from build123d import *

# Parameters (mm, degrees)
F1_DEPTH = 25.4
F3_D     = 4.318
F3_DEPTH = 5.08
F3_TIP   = 1.2972580765
F5_D     = 2.9464
F5_DEPTH = 5.08
F5_TIP   = 0.885187864


with BuildPart() as f1:
    # F0 (on Front) → F1 (new body)
    with BuildSketch(Plane.XZ):
        with BuildLine():
            ThreePointArc((-3.175, 0), (-0.9299359697, 0.9299359697), (0, 3.175))
            Line((0, 3.175), (0, 31.75))
            Line((0, 31.75), (-3.175, 31.75))
            Line((-3.175, 31.75), (-3.175, 6.35))
            ThreePointArc((-3.175, 6.35), (-4.1049359697, 4.1049359697), (-6.35, 3.175))
            Line((-6.35, 3.175), (-22.225, 3.175))
            Line((-22.225, 3.175), (-22.225, 0))
            Line((-22.225, 0), (-3.175, 0))
        make_face()
    extrude(amount=F1_DEPTH)

    # F3
    with Locations(Plane(origin=(-3.175, 0, 0), x_dir=(0, -1, 0), z_dir=(-1, 0, 0))):
        with Locations((6.35, 12.7), (6.35, 25.4), (19.05, 25.4), (19.05, 12.7)):
            Hole(F3_D / 2, depth=F3_DEPTH)
            with Locations((0, 0, -(F3_DEPTH + F3_TIP / 2))):  # 118° drill point
                Cone(0, F3_D / 2, F3_TIP, mode=Mode.SUBTRACT)

    # F5
    with Locations(Plane(origin=(0, 0, 0), x_dir=(1, 0, 0), z_dir=(0, 0, -1))):
        with Locations((-6.35, 6.35), (-6.35, 19.05), (-15.875, 19.05), (-15.875, 6.35)):
            Hole(F5_D / 2, depth=F5_DEPTH)
            with Locations((0, 0, -(F5_DEPTH + F5_TIP / 2))):  # 118° drill point
                Cone(0, F5_D / 2, F5_TIP, mode=Mode.SUBTRACT)


solid = f1.part
Work out the finished part from the listing and answer in its coordinate system (mm). A direction names the side the tool comes from. Round coordinates to 2 decimals unless told otherwise and drop trailing zeros. Loops run counter-clockwise (first coordinate to the right, second up) from the corner with the lowest first, then second, coordinate; pieces in that order, holes last. Notation, with made-up numbers: (66, -10.5) - (71, -10.5) arc R20 cw to (71, 7.5) - close; hole circle Ø4 at (53.25, 75). An arc over 180 degrees is marked (long way). Use one line per item in the form item = value. Start each with the question number.
(1) Consider line 1 (Y direction, x = -6.35, z = 2); line 2 (Z direction, x = -0.9, y = -19.05); line 3 (Y direction, x = -1.75, z = 26.5). Determine where each line is inside the solid, lowest interval first.
(2) Find section C-C on y = -22.75. Determine the outline of the cut face in (x, z) (3 decimals).
(3) Which of the six approach directions +Z, -Z, +X, -X, +Y, -Y give full straight-line access (tool end or side, diameter ignored) to faces 1 (the face through (-17.28, -6.79, 1.61)), 2 (the face through (-14, -13, 3.175))?
(4) Find section D-D on x = -13.5. Determine the outline of the cut face in (y, z) (3 decimals).
(5) Flat-ended cylindrical pins translate along their axes: P1, Ø1.5, axis at x = -17.5, z = 4.5, coming from the +Y side; P2, Ø7, axis at y = -6.35, z = 12.7, coming from the -X side (3 decimals); P3, Ø3.5, axis at x = -15.875, y = -19.05, coming from the -Z side. Find the tip coordinate at first contact, or state that the pin passes through.
(6) Determine the mould class of faces 3 (the face through (-4.08, -12.52, 4.13)), 4 (the face through (-3.175, -13, 19)), 5 (the face through (-1.565, -19.518, 10.592)), 6 (the face through (-0.95, -12.52, 0.91)) for opening direction Z: +Z half, -Z half, draft (parallel to the pull), parting line (faces both ways), or undercut.
(7) Find section A-A on y = -19.05. Determine the outline of the cut face in (x, z) (3 decimals).
(8) Find section B-B on z = 12.7. Determine the outline of the cut face in (x, y) (3 decimals), and give its area (3 significant figures).
Answer list:
q1.line_1 = -25.4 to -20.52, -17.58 to -7.82, -4.88 to 0
q1.line_2 = 0.96 to 10.54, 14.86 to 23.24, 27.56 to 31.75
q1.line_3 = -25.4 to -20.91, -17.19 to -8.21, -4.49 to 0
q2.outline = (-22.225, 0) - (-3.175, 0) arc R3.175 ccw to (0, 3.175) - (0, 31.75) - (-3.175, 31.75) - (-3.175, 6.35) arc R3.175 cw to (-6.35, 3.175) - (-22.225, 3.175) - close
q3.face_1 = +Z, -Z
q3.face_2 = +Z, -X, +Y, -Y
q4.outline = (-25.4, 0) - (0, 0) - (0, 3.175) - (-25.4, 3.175) - close
q5.P1 = through
q5.P2 = -3.175
q5.P3 = 0
q6.face_3 = +Z half
q6.face_4 = draft
q6.face_5 = undercut
q6.face_6 = -Z half
q7.outline = (-22.225, 0) - (-17.348, 0) - (-17.348, 3.175) - (-22.225, 3.175) - close; (-14.402, 0) - (-7.823, 0) - (-7.823, 3.175) - (-14.402, 3.175) - close; (-4.877, 0) - (-3.175, 0) arc R3.175 ccw to (0, 3.175) - (0, 10.541) - (-3.175, 10.541) - (-3.175, 6.35) arc R3.175 cw to (-4.877, 3.537) - close; (-3.175, 14.859) - (0, 14.859) - (0, 23.241) - (-3.175, 23.241) - close; (-3.175, 27.559) - (0, 27.559) - (0, 31.75) - (-3.175, 31.75) - close
q8.outline = (-3.175, -25.4) - (0, -25.4) - (0, -21.209) - (-3.175, -21.209) - close; (-3.175, -16.891) - (0, -16.891) - (0, -8.509) - (-3.175, -8.509) - close; (-3.175, -4.191) - (0, -4.191) - (0, 0) - (-3.175, 0) - close
q8.area = 53.2 mm^2
